```python
from build123d import *

# Parameters (mm, degrees)
CROQUIS1_R              = 15
CROQUIS1_R_2            = 2.25
SALIENTE_EXTRUIR1_DEPTH = 2
CROQUIS3_R              = 5
CROQUIS3_R_2            = 2.25
SALIENTE_EXTRUIR2_DEPTH = 8.5
CROQUIS4_R              = 3.75
CORTAR_EXTRUIR1_DEPTH   = 4


with BuildPart() as part:
    # Croquis1 → Saliente-Extruir1 (new body)
    with BuildSketch(Plane(origin=(0, 0, 0), x_dir=(0, 0, -1), z_dir=(1, 0, 0))):
        Circle(CROQUIS1_R)
        Circle(CROQUIS1_R_2, mode=Mode.SUBTRACT)
    extrude(amount=SALIENTE_EXTRUIR1_DEPTH)

    # Croquis3 → Saliente-Extruir2 (add)
    with BuildSketch(Plane(origin=(2, 0, 0), x_dir=(0, 0, -1), z_dir=(1, 0, 0))):
        Circle(CROQUIS3_R)
        Circle(CROQUIS3_R_2, mode=Mode.SUBTRACT)
    extrude(amount=SALIENTE_EXTRUIR2_DEPTH)

    # Croquis4 → Cortar-Extruir1 (cut)
    with BuildSketch(Plane.ZY):
        Circle(CROQUIS4_R)
    extrude(amount=-CORTAR_EXTRUIR1_DEPTH, mode=Mode.SUBTRACT)


solid = part.part
```
Read the model definition and answer for the solid it produces. Units are mm, in the model's axes. A direction names the side the tool comes from. Round coordinates to 2 decimals unless told otherwise and drop trailing zeros. Loops run counter-clockwise (first coordinate to the right, second up) from the corner with the lowest first, then second, coordinate; pieces in that order, holes last. Notation, with made-up numbers: (33, -4) -> (73, -4) arc R21 cw to (73, 26) -> close; hole circle Ø10 at (53, -16.75). An arc over 180 degrees is marked (long way). One line per item, written item: value.
1) The mould has two halves that part along Z. Classify faces 4 (the face through (7.2, 2.23, 0.29)), 5 (the face through (0, -3, -3)), 6 (the face through (0.986, 0.66, 14.985)), 7 (the face through (4, -2, 2)): pulls with the +Z half, pulls with the -Z half, needs draft (parallel to the pull), parting line crosses it, or undercut.
Answer list:
face 4: undercut
face 5: needs draft
face 6: parting line crosses it
face 7: undercut
2) For faces 1 (the face through (6.19, -4.88, 1.08)), 2 (the face through (1.972, 0.165, -3.746)), 3 (the face through (10.5, -1, -2.2)), determine the directions among +Z, -Z, +X, -X, +Y, -Y from which every point of the face is accessible in a straight line to the end or side of a thin tool.
Answer list:
face 1: +X
face 2: -X
face 3: +Z, -Z, +X, +Y, -Y
3) Flat-ended cylindrical pins translate along their axes: P1, Ø7, axis at y = 0, z = 0, coming from the -X side; P2, Ø6, axis at x = 1, z = -11.5, coming from the +Y side; P3, Ø1, axis at x = 2, z = -10.5, coming from the -Y side. Find the tip coordinate at first contact, or state that the pin passes through.
Answer list:
P1: stops at x = 4
P2: stops at y = 12.36
P3: stops at y = -11.18
4) A cutting plane is placed at D-D (y = -12). Determine the outline of the cut face in (x, z).
Answer list:
outline: (0, -9) -> (2, -9) -> (2, 9) -> (0, 9) -> close
5) A cutting plane is placed at A-A (z = 0). Determine the outline of the cut face in (x, y).
Answer list:
outline: (0, -15) -> (2, -15) -> (2, -5) -> (10.5, -5) -> (10.5, -2.25) -> (4, -2.25) -> (4, -3.75) -> (0, -3.75) -> close; (0, 3.75) -> (4, 3.75) -> (4, 2.25) -> (10.5, 2.25) -> (10.5, 5) -> (2, 5) -> (2, 15) -> (0, 15) -> close
6) Consider L1, parallel to Y at x = 3, z = 0; L2, parallel to X at y = -5.5, z = 4.75; L3, parallel to Y at x = 7.25, z = 0. Determine where each line is inside the solid, lowest interval first. Write a range as [from, to].
Answer list:
L1: y = [-5, -3.75], [3.75, 5]
L2: x = [0, 2]
L3: y = [-5, -2.25], [2.25, 5]
7) A cutting plane is placed at C-C (x = 7.5). Determine the outline of the cut face in (y, z), and give its area (3 significant figures).
Answer list:
outline: circle Ø10 at (0, 0); hole circle Ø4.5 at (0, 0)
area: 62.6 mm²
